Could you check a few things on this model? Use its own coordinates, in mm. Face numbers are marked on the shaded views. A direction names the side the tool comes from. Give positions to 0.01 mm unless a question says otherwise; leave off trailing zeros. Order: outer loops, then holes, each group sorted by start corner. A loop starts at its lowest first (then second) coordinate and runs counter-clockwise, first axis right, second up. Notation, with made-up numbers: (-18.75, 40) - (-3.75, 40) arc R22 cw to (-3.75, 54) - close; hole circle Ø3 at (37.25, 69). An arc over 180 degrees is marked (long way). Put each result on its own line as item: value.
from build123d import *

# Parameters (mm, degrees)
SKETCH1_R                           = 25.4
BOSS_EXTRUDE1_DEPTH                 = 25.4
SKETCH2_R                           = 16
CUT_EXTRUDE1_DEPTH                  = 21.59
CUT_EXTRUDE2_REACH                  = 45.994
CUT_EXTRUDE2_END_RADIUS             = 25.4
SKETCH3_W                           = 3.81
SKETCH3_H                           = 16.51
CUT_EXTRUDE2_DIRECTION_2_REACH      = 45.994
CUT_EXTRUDE2_DIRECTION_2_END_RADIUS = 25.4
CUT_EXTRUDE3_REACH                  = 43.91
SKETCH4_R                           = 1


with BuildPart() as part:
    # Sketch1 → Boss-Extrude1 (new body)
    with BuildSketch(Plane(origin=(0, 0, 0), x_dir=(1, 0, 0), z_dir=(0, 1, 0))):
        with Locations(Location((0, 0, 0), (0, 0, 270))):
            Circle(SKETCH1_R)
    extrude(amount=BOSS_EXTRUDE1_DEPTH)

    # Sketch2 → Cut-Extrude1 (cut)
    with BuildSketch(Plane(origin=(0, 25.4, 0), x_dir=(1, 0, 0), z_dir=(0, 1, 0))):
        with Locations(Location((0, 0, 0), (0, 0, 270))):
            Circle(SKETCH2_R)
    extrude(amount=-CUT_EXTRUDE1_DEPTH, mode=Mode.SUBTRACT)

    # Cut-Extrude2: up to this cylinder (the profile starts inside it)
    cut_extrude2_end = Plane(origin=(0, 17.145, 0), z_dir=(0, -1, 0)) * Cylinder(CUT_EXTRUDE2_END_RADIUS, 143.788, mode=Mode.PRIVATE)
    # Sketch3 → Cut-Extrude2 (cut, up to the surface)
    with BuildSketch(Plane.XY, mode=Mode.PRIVATE) as cut_extrude2_sk1:
        with Locations((23.495, 17.145)):
            Rectangle(SKETCH3_W, SKETCH3_H)
    cut_extrude2_tool1 = extrude(cut_extrude2_sk1.sketch, amount=-CUT_EXTRUDE2_REACH, mode=Mode.PRIVATE) & cut_extrude2_end
    add(cut_extrude2_tool1.solids().sort_by_distance((23.495, 17.145, 0))[0], mode=Mode.SUBTRACT)
    # Sketch3 → Cut-Extrude2 (cut, up to the surface)
    with BuildSketch(Plane.XY, mode=Mode.PRIVATE) as cut_extrude2_sk2:
        with Locations((-23.495, 17.145)):
            Rectangle(SKETCH3_W, SKETCH3_H)
    cut_extrude2_tool2 = extrude(cut_extrude2_sk2.sketch, amount=-CUT_EXTRUDE2_REACH, mode=Mode.PRIVATE) & cut_extrude2_end
    add(cut_extrude2_tool2.solids().sort_by_distance((-23.495, 17.145, 0))[0], mode=Mode.SUBTRACT)

    # Cut-Extrude2 direction 2: up to this cylinder (the profile starts inside it)
    cut_extrude2_direction_2_end = Plane(origin=(0, 17.145, 0), z_dir=(0, -1, 0)) * Cylinder(CUT_EXTRUDE2_DIRECTION_2_END_RADIUS, 143.788, mode=Mode.PRIVATE)
    # Sketch3 → Cut-Extrude2 direction 2 (cut, up to the surface)
    with BuildSketch(Plane.XY, mode=Mode.PRIVATE) as cut_extrude2_direction_2_sk1:
        with Locations((23.495, 17.145)):
            Rectangle(SKETCH3_W, SKETCH3_H)
    cut_extrude2_direction_2_tool1 = extrude(cut_extrude2_direction_2_sk1.sketch, amount=CUT_EXTRUDE2_DIRECTION_2_REACH, mode=Mode.PRIVATE) & cut_extrude2_direction_2_end
    add(cut_extrude2_direction_2_tool1.solids().sort_by_distance((23.495, 17.145, 0))[0], mode=Mode.SUBTRACT)
    # Sketch3 → Cut-Extrude2 direction 2 (cut, up to the surface)
    with BuildSketch(Plane.XY, mode=Mode.PRIVATE) as cut_extrude2_direction_2_sk2:
        with Locations((-23.495, 17.145)):
            Rectangle(SKETCH3_W, SKETCH3_H)
    cut_extrude2_direction_2_tool2 = extrude(cut_extrude2_direction_2_sk2.sketch, amount=CUT_EXTRUDE2_DIRECTION_2_REACH, mode=Mode.PRIVATE) & cut_extrude2_direction_2_end
    add(cut_extrude2_direction_2_tool2.solids().sort_by_distance((-23.495, 17.145, 0))[0], mode=Mode.SUBTRACT)

    # Sketch4 → Cut-Extrude3 (cut, up to next)
    with BuildSketch(Plane(origin=(0, 3.81, 0), x_dir=(1, 0, 0), z_dir=(0, 1, 0)), mode=Mode.PRIVATE) as cut_extrude3_sk1:
        with Locations(Location((0, 8.89, 0), (0, 0, 270))):
            Circle(SKETCH4_R)
    cut_extrude3_tool1 = extrude(cut_extrude3_sk1.sketch, amount=-CUT_EXTRUDE3_REACH, mode=Mode.PRIVATE) & part.part
    # Sketch4 → Cut-Extrude3 (cut, up to next)
    with BuildSketch(Plane(origin=(0, 3.81, 0), x_dir=(1, 0, 0), z_dir=(0, 1, 0)), mode=Mode.PRIVATE) as cut_extrude3_sk2:
        with Locations(Location((7.69896584, -4.445, 0), (0, 0, 270))):
            Circle(SKETCH4_R)
    cut_extrude3_tool2 = extrude(cut_extrude3_sk2.sketch, amount=-CUT_EXTRUDE3_REACH, mode=Mode.PRIVATE) & part.part
    # Sketch4 → Cut-Extrude3 (cut, up to next)
    with BuildSketch(Plane(origin=(0, 3.81, 0), x_dir=(1, 0, 0), z_dir=(0, 1, 0)), mode=Mode.PRIVATE) as cut_extrude3_sk3:
        with Locations(Location((-7.69896584, -4.445, 0), (0, 0, 270))):
            Circle(SKETCH4_R)
    cut_extrude3_tool3 = extrude(cut_extrude3_sk3.sketch, amount=-CUT_EXTRUDE3_REACH, mode=Mode.PRIVATE) & part.part
    add(cut_extrude3_tool1.solids().sort_by_distance((0, 3.81, -8.89))[0], mode=Mode.SUBTRACT)
    add(cut_extrude3_tool2.solids().sort_by_distance((7.698966, 3.81, 4.445))[0], mode=Mode.SUBTRACT)
    add(cut_extrude3_tool3.solids().sort_by_distance((-7.698966, 3.81, 4.445))[0], mode=Mode.SUBTRACT)


solid = part.part
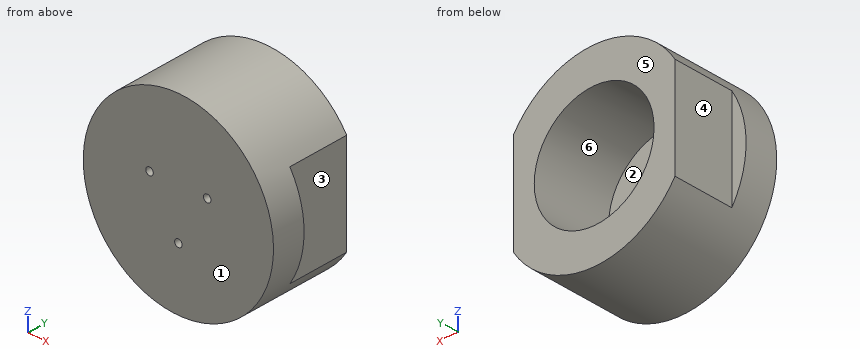
1) Suppose I cut it at B-B, the plane y = 20.25. List the corners of the cut face in (x, z) for me, and give its area (3 significant figures).
Filled in:
outline: (-21.59, -13.38) arc R25.4 ccw to (21.59, -13.38) - (21.59, 13.38) arc R25.4 ccw to (-21.59, 13.38) - close; hole circle Ø32 at (0, 0)
area: 1,080 mm^2
2) Suppose I cut it at D-D, the plane z = -8.89. List the corners of the cut face in (x, y) for me, and give its area (3 significant figures).
Filled in:
outline: (-23.79, 0) - (-1, 0) - (-1, 3.81) - (-13.3, 3.81) - (-13.3, 25.4) - (-21.59, 25.4) - (-21.59, 8.89) - (-23.79, 8.89) - close; (1, 0) - (23.79, 0) - (23.79, 8.89) - (21.59, 8.89) - (21.59, 25.4) - (13.3, 25.4) - (13.3, 3.81) - (1, 3.81) - close
area: 554 mm^2
3) Suppose I cut it at A-A, the plane x = 0. List the corners of the cut face in (y, z) for me, and give its area (3 significant figures).
Filled in:
outline: (0, -25.4) - (25.4, -25.4) - (25.4, -16) - (3.81, -16) - (3.81, -9.89) - (0, -9.89) - close; (0, -7.89) - (3.81, -7.89) - (3.81, 16) - (25.4, 16) - (25.4, 25.4) - (0, 25.4) - close
area: 592 mm^2
4) Suppose I cut it at C-C, the plane z = 0. List the corners of the cut face in (x, y) for me, and give its area (3 significant figures).
Filled in:
outline: (-25.4, 0) - (25.4, 0) - (25.4, 8.89) - (21.59, 8.89) - (21.59, 25.4) - (16, 25.4) - (16, 3.81) - (-16, 3.81) - (-16, 25.4) - (-21.59, 25.4) - (-21.59, 8.89) - (-25.4, 8.89) - close
area: 474 mm^2
5) If I drill on line 1 (X direction, y = 11, z = 0); line 2 (Z direction, x = -14, y = 15); line 3 (Z direction, x = 1.5, y = 13.25), over which ranges is the centre line in solid material (lowest first)? Write a range as [from, to].
Filled in:
line 1: x = [-21.59, -16], [16, 21.59]
line 2: z = [-21.19, -7.75], [7.75, 21.19]
line 3: z = [-25.36, -15.93], [15.93, 25.36]
6) Which directions (+Z, -Z, +X, -X, +Y, -Y) give clear straight access to the entire face, cutting with the end or side of a thin tool? Please do the marked faces 1, 2 and 3.
Filled in:
face 1: +Z, -Z, +X, -X, -Y
face 2: +Y
face 3: +Z, -Z, +X, +Y
7) We'd pull the mould along X, two halves only. Please class the marked faces 4, 5 and 6: pulls with the +X half, pulls with the -X half, needs draft (parallel to the pull), parting line crosses it, or undercut.
Filled in:
face 4: pulls with the -X half
face 5: needs draft
face 6: undercut
8) I'm going to push flat-ended pins straight in: pin 1 (2.5 mm diameter, centred on x = -7.7, z = 4.44, fed in from +Y); pin 2 (10 mm diameter, centred on y = 15.5, z = -10.5, fed in from -X); pin 3 (1.1 mm diameter, centred on x = 23.5, z = -4.5, fed in from +Y). Where does each tip first touch, or does it pass through?
Filled in:
pin 1: stops at y = 3.81
pin 2: stops at x = -21.59
pin 3: stops at y = 8.89
